Read the model definition and answer for the solid it produces. Units are mm, in the model's axes. Face numbers are marked on the shaded views. A direction names the side the tool comes from. Give positions to 0.01 mm unless a question says otherwise; leave off trailing zeros. Write each loop counter-clockwise with the first axis right and the second up, starting at its lowest first coordinate (ties: lowest second). Pieces come first, ordered by that corner, then holes. Notation, with made-up numbers: (-18.5, -30.75) -> (17.5, -30.75) arc R25 ccw to (17.5, 6.25) -> close; hole circle Ø4 at (71.25, 65.25). An arc over 180 degrees is marked (long way). Use a Markdown table: item, result.
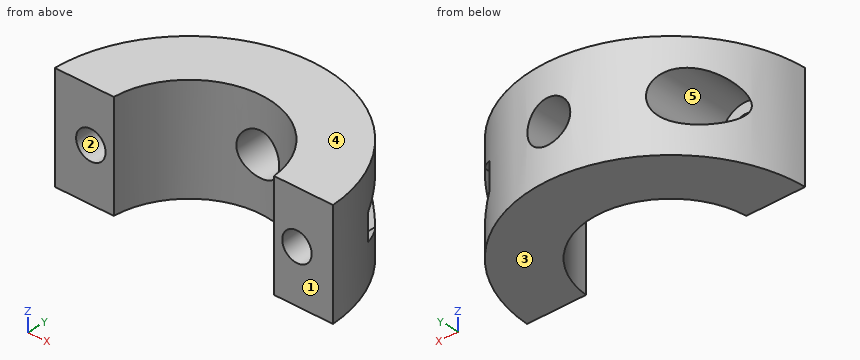
from build123d import *

# Parameters (mm, degrees)
PAD_DEPTH       = 20
SKETCH001_R     = 2.75
SKETCH001_R_2   = 4
POCKET_DEPTH    = 25.001
SKETCH002_R     = 4.75
POCKET001_DEPTH = 20.001


with BuildPart() as part:
    # Sketch → Pad (new body)
    with BuildSketch(Plane.XY):
        with BuildLine():
            ThreePointArc((14.96663, 0), (0, 14), (-14.96663, 0))
            Line((-25.980762, 0), (-14.96663, 0))
            ThreePointArc((25.980762, 0), (0, 25), (-25.980762, 0))
            Line((14.96663, 0), (25.980762, 0))
        make_face()
    extrude(amount=PAD_DEPTH)

    # Sketch001 (on Face2 of Pad) → Pocket (cut, through all)
    with BuildSketch(Plane.XZ):
        with Locations((-19.25, 10)):
            Circle(SKETCH001_R)
        with Locations((19.25, 10)):
            Circle(SKETCH001_R)
        with Locations((0, 10)):
            Circle(SKETCH001_R_2)
    extrude(amount=-POCKET_DEPTH, mode=Mode.SUBTRACT)

    # Sketch002 (on DatumPlane) → Pocket001 (cut, through all)
    with BuildSketch(Plane.XZ.offset(-5)):
        with Locations((-19.25, 10)):
            Circle(SKETCH002_R)
        Polygon((19.25, 5.092523), (23.5, 7.546261), (23.5, 12.453739), (19.25, 14.907477), (15, 12.453739), (15, 7.546261), align=None)
    extrude(amount=-POCKET001_DEPTH, mode=Mode.SUBTRACT)


solid = part.part
Item 1: A cutting plane is placed at D-D (z = 17.5). Give the vertices of the cut face in (x, y), then the cut area to 3 significant figures.
Return value:
| item | result |
|---|---|
| outline | (-25.98, 0) -> (-14.97, 0) arc R15 cw to (14.97, 0) -> (25.98, 0) arc R26 ccw to start |
| area | 686 mm^2 |
Item 2: Each of these flat-tipped pins is pushed along its axis until it touches: P1, Ø9.5, axis at x = 18, z = 11.5, coming from the +Y side; P2, Ø3, axis at x = 2.5, z = 4, coming from the -Y side; P3, Ø2, axis at y = 9.5, z = 16, coming from the +X side; P4, Ø8, axis at x = -18, y = 14.5, coming from the -Z side. Where does it stop, or does it pass through?
Return value:
| item | result |
|---|---|
| P1 | y = 21.37 |
| P2 | y = 13.46 |
| P3 | x = 24.2 |
| P4 | z = 0 |
Item 3: A cutting plane is placed at B-B (z = 9.25). Give the vertices of the cut face in (x, y).
Return value:
| item | result |
|---|---|
| outline | (-25.98, 0) -> (-21.9, 0) -> (-21.9, 5) -> (-23.94, 5) -> (-23.94, 9.14) arc R26 ccw to start; (-16.6, 0) -> (-14.97, 0) arc R15 cw to (-3.93, 13.48) -> (-3.93, 24.7) arc R26 ccw to (-14.56, 20.54) -> (-14.56, 5) -> (-16.6, 5) -> close; (3.93, 13.48) arc R15 cw to (14.97, 0) -> (16.6, 0) -> (16.6, 5) -> (15, 5) -> (15, 20.24) arc R26 ccw to (3.93, 24.7) -> close; (21.9, 0) -> (25.98, 0) arc R26 ccw to (23.5, 10.12) -> (23.5, 5) -> (21.9, 5) -> close |
Item 4: A cutting plane is placed at A-A (x = -19.25). Give the vertices of the cut face in (y, z).
Return value:
| item | result |
|---|---|
| outline | (0, 0) -> (16.48, 0) -> (16.48, 5.25) -> (5, 5.25) -> (5, 7.25) -> (0, 7.25) -> close; (0, 12.75) -> (5, 12.75) -> (5, 14.75) -> (16.48, 14.75) -> (16.48, 20) -> (0, 20) -> close |
Item 5: Straight lines are drawn through the part: line 1 along Z through (x, y) = (19.25, 2.25); line 2 along Y through (x, z) = (16.5, 12); line 3 along Z through (x, y) = (16, 8.5). For each, find the intervals that lie inside material, in ascending order. Write a range as [from, to].
Return value:
| item | result |
|---|---|
| line 1 | [0, 7.25], [12.75, 20] |
| line 2 | [0, 5] |
| line 3 | [0, 6.97], [13.03, 20] |
Item 6: A tool of negligible diameter and unlimited length cuts with its end or side. For the marked faces 4 and 5, from which of +Z, -Z, +X, -X, +Y, -Y can it reach the whole face along a straight path? Write none if from no direction.
Return value:
| item | result |
|---|---|
| face 4 | +Z, +X, -X, +Y, -Y |
| face 5 | +Y |
Item 7: For a pull along Z with two mould halves and no side action, classify the marked faces 1, 2 and 3 as +Z half, -Z half, draft (parallel to the pull), parting line (faces both ways), or undercut.
Return value:
| item | result |
|---|---|
| face 1 | draft |
| face 2 | undercut |
| face 3 | -Z half |
Item 8: A cutting plane is placed at C-C (x = 0). Give the vertices of the cut face in (y, z).
Return value:
| item | result |
|---|---|
| outline | (14, 0) -> (25, 0) -> (25, 6) -> (14, 6) -> close; (14, 14) -> (25, 14) -> (25, 20) -> (14, 20) -> close |
